CAD build for the part. Positions are in the model's coordinates, mm. A direction names the side the tool comes from. Round coordinates to 2 decimals unless told otherwise and drop trailing zeros. Write each loop counter-clockwise with the first axis right and the second up, starting at its lowest first coordinate (ties: lowest second). Pieces come first, ordered by that corner, then holes. Notation, with made-up numbers: (12.25, 78.25) - (24.25, 78.25) arc R16 cw to (24.25, 103.25) - close; hole circle Ø9 at (41.25, -9). An arc over 180 degrees is marked (long way). Answer in a Markdown table with one row per item.
```python
from build123d import *
from build123d.topology import SkipClean

# Parameters (mm, degrees)
CROQUIS1_R                        = 35
CROQUIS1_R_2                      = 4.75
SALIENTE_EXTRUIR1_DEPTH           = 3
CROQUIS2_R                        = 1.95
SALIENTE_EXTRUIR2_DEPTH           = 5
SALIENTE_EXTRUIR3_START           = 1
CROQUIS5_R                        = 2.25
SALIENTE_EXTRUIR3_DEPTH           = 4
SALIENTE_EXTRUIR3_DRAFT           = 4
SALIENTE_EXTRUIR3_PROFILE_2_DEPTH = 4
SALIENTE_EXTRUIR3_PROFILE_2_DRAFT = 4
CROQUIS3_W                        = 1
CROQUIS3_H                        = 6.840682912
CORTAR_EXTRUIR1_DEPTH             = 4
CROQUIS6_W                        = 5.727241663
CROQUIS6_H                        = 1.622786798
CROQUIS6_W_2                      = 5.017003251
CROQUIS6_H_2                      = 0.546869116
CROQUIS6_W_3                      = 4.668475527
CROQUIS6_H_3                      = 1.179349449
CROQUIS6_W_4                      = 4.588943699
CROQUIS6_H_4                      = 1.521824685
CORTAR_EXTRUIR2_DEPTH             = 4
SALIENTE_EXTRUIR4_START           = 35
SALIENTE_EXTRUIR4_DEPTH           = 35
CROQUIS9_W                        = 86.6
CROQUIS9_H                        = 71.3
SALIENTE_EXTRUIR5_DEPTH           = 3
CROQUIS10_W                       = 86.6
CROQUIS10_H                       = 71.3
CROQUIS10_W_2                     = 80.6
CROQUIS10_H_2                     = 65.3
SALIENTE_EXTRUIR6_DEPTH           = 32
CORTAR_EXTRUIR3_REACH             = 106.595
CROQUIS11_W                       = 40
CROQUIS11_H                       = 3
CROQUIS12_R                       = 2.5
CROQUIS12_R_2                     = 1.59
SALIENTE_EXTRUIR7_DEPTH           = 5
CROQUIS13_W                       = 14
CROQUIS13_H                       = 14
CROQUIS13_W_2                     = 11
CROQUIS13_H_2                     = 11
CORTAR_EXTRUIR4_DEPTH             = 3


with BuildPart() as part:
    # Croquis1 → Saliente-Extruir1 (new body)
    with BuildSketch(Plane(origin=(0, 0, 0), x_dir=(1, 0, 0), z_dir=(0, 1, 0))):
        with Locations(Location((0, 0, 0), (0, 0, 270))):
            Circle(CROQUIS1_R)
        with Locations(Location((0, 0, 0), (0, 0, 270))):
            Circle(CROQUIS1_R_2, mode=Mode.SUBTRACT)
    extrude(amount=SALIENTE_EXTRUIR1_DEPTH)

    # Croquis2 → Saliente-Extruir2 (add)
    with BuildSketch(Plane.XZ):
        with Locations(Location((-17.5, 8, 0), (0, 0, 90))):
            Circle(CROQUIS2_R)
        with Locations(Location((17.5, 8, 0), (0, 0, 90))):
            Circle(CROQUIS2_R)
    extrude(amount=SALIENTE_EXTRUIR2_DEPTH)


with BuildPart() as saliente_extruir3_tool:
    # Croquis5 → Saliente-Extruir3 (with draft: the straight prism first)
    with BuildSketch(Plane.XZ.offset(SALIENTE_EXTRUIR3_START)):
        with Locations((-17.5, 8)):
            Circle(CROQUIS5_R)
    extrude(amount=SALIENTE_EXTRUIR3_DEPTH)
    # Saliente-Extruir3: the draft: its side faces are tilted about the plane it starts from
    saliente_extruir3_sides = [saliente_extruir3_tool.faces().sort_by_distance(p)[0] for p in [
        (-19.75, -3, 8),
    ]]
    draft(saliente_extruir3_sides, Plane.XZ.offset(SALIENTE_EXTRUIR3_START), SALIENTE_EXTRUIR3_DRAFT)


with BuildPart() as part_1:
    add(part.part)

    # Saliente-Extruir3: add saliente_extruir3_tool
    add(saliente_extruir3_tool.part)


with BuildPart() as saliente_extruir3_profile_2_tool:
    # Croquis5 → Saliente-Extruir3 profile 2 (with draft: the straight prism first)
    with BuildSketch(Plane.XZ.offset(SALIENTE_EXTRUIR3_START)):
        with Locations((17.5, 8)):
            Circle(CROQUIS5_R)
    extrude(amount=SALIENTE_EXTRUIR3_PROFILE_2_DEPTH)
    # Saliente-Extruir3 profile 2: the draft: its side faces are tilted about the plane it starts from
    saliente_extruir3_profile_2_sides = [saliente_extruir3_profile_2_tool.faces().sort_by_distance(p)[0] for p in [
        (15.25, -3, 8),
    ]]
    draft(saliente_extruir3_profile_2_sides, Plane.XZ.offset(SALIENTE_EXTRUIR3_START), SALIENTE_EXTRUIR3_PROFILE_2_DRAFT)


with BuildPart() as part_2:
    add(part_1.part)

    # Saliente-Extruir3 profile 2: add saliente_extruir3_profile_2_tool
    add(saliente_extruir3_profile_2_tool.part)

    # Croquis3 → Cortar-Extruir1 (cut)
    with BuildSketch(Plane.XZ.offset(5)):
        with Locations((-17.5, 7.675365729)):
            Rectangle(CROQUIS3_W, CROQUIS3_H)
        with Locations((17.5, 7.675365729)):
            Rectangle(CROQUIS3_W, CROQUIS3_H)
    extrude(amount=-CORTAR_EXTRUIR1_DEPTH, mode=Mode.SUBTRACT)

    # Croquis6 → Cortar-Extruir2 (cut)
    with BuildSketch(Plane.XZ.offset(1)):
        with Locations((-17.258839661, 10.696201081)):
            Rectangle(CROQUIS6_W, CROQUIS6_H)
        with Locations((-17.417509945, 5.84175776)):
            Rectangle(CROQUIS6_W_2, CROQUIS6_H_2)
        with Locations((17.632507556, 10.474482406)):
            Rectangle(CROQUIS6_W_3, CROQUIS6_H_3)
        with Locations((17.310781188, 5.354279976)):
            Rectangle(CROQUIS6_W_4, CROQUIS6_H_4)
    extrude(amount=CORTAR_EXTRUIR2_DEPTH, mode=Mode.SUBTRACT)

    # Croquis7 → Saliente-Extruir4 (add)
    with SkipClean():  # the faces are left unmerged after this step: merging them gives an invalid solid
        with BuildSketch(Plane.XZ.offset(SALIENTE_EXTRUIR4_START)):
            with BuildLine():
                Line((-22.651194874, 22.651194874), (-24.748737342, 24.748737342))
                ThreePointArc((-24.748737342, 24.748737342), (-15.674335611, 31.294012257), (-4.998139738, 34.641284606))
                Line((-4.998139738, 34.641284606), (-4.998139738, 31.641284606))
                ThreePointArc((-4.998139738, 31.641284606), (-14.537086186, 28.545154562), (-22.651194874, 22.651194874))
            make_face()
            with BuildLine():
                Line((22.651200534, 22.651200534), (24.748737342, 24.748737342))
                ThreePointArc((24.748737342, 24.748737342), (15.675128347, 31.293615184), (4.999894801, 34.641031335))
                Line((4.999894801, 34.641031335), (4.999894801, 31.641031335))
                ThreePointArc((4.999894801, 31.641031335), (14.537881979, 28.544766366), (22.651200534, 22.651200534))
            make_face()
        extrude(amount=-SALIENTE_EXTRUIR4_DEPTH)

    # Croquis9 → Saliente-Extruir5 (add)
    with SkipClean():  # the faces are left unmerged after this step: merging them gives an invalid solid
        with BuildSketch(Plane.XZ):
            with Locations((0, -51.65)):
                Rectangle(CROQUIS9_W, CROQUIS9_H)
        extrude(amount=SALIENTE_EXTRUIR5_DEPTH)

    # Croquis10 → Saliente-Extruir6 (add)
    with SkipClean():  # the faces are left unmerged after this step: merging them gives an invalid solid
        with BuildSketch(Plane.XZ.offset(3)):
            with Locations((0, -51.65)):
                Rectangle(CROQUIS10_W, CROQUIS10_H)
            with Locations((0, -51.65)):
                Rectangle(CROQUIS10_W_2, CROQUIS10_H_2, mode=Mode.SUBTRACT)
        extrude(amount=SALIENTE_EXTRUIR6_DEPTH)

    # Cortar-Extruir3: up to this face of the body (flat: up to its plane)
    cortar_extruir3_end = Plane(part_2.part.faces().sort_by_distance((1.0887e-05, 0, 5.820345138))[0])
    # Croquis11 → Cortar-Extruir3 (cut, up to the picked face)
    with BuildSketch(Plane.XZ.offset(35), mode=Mode.PRIVATE) as cortar_extruir3_sk1:
        with Locations((0, -17.5)):
            Rectangle(CROQUIS11_W, CROQUIS11_H)
    cortar_extruir3_tool1 = split(extrude(cortar_extruir3_sk1.sketch, amount=-CORTAR_EXTRUIR3_REACH, mode=Mode.PRIVATE), bisect_by=cortar_extruir3_end, keep=Keep.BOTH, mode=Mode.PRIVATE)
    add(cortar_extruir3_tool1.solids().sort_by(Axis((0, -35, -17.5), (0, 1, 0)))[0], mode=Mode.SUBTRACT)

    # Croquis12 → Saliente-Extruir7 (add)
    # profile 1 of 4: a face of its own
    with SkipClean():  # the faces are left unmerged after this step: merging them gives an invalid solid
        with BuildSketch(Plane.XZ.offset(3)):
            with Locations(Location((31.8, -42.7, 0), (0, 0, 270))):
                Circle(CROQUIS12_R)
            with Locations(Location((31.8, -42.7, 0), (0, 0, 270))):
                Circle(CROQUIS12_R_2, mode=Mode.SUBTRACT)
        # profile 2 of 4: a face of its own
        with BuildSketch(Plane.XZ.offset(3)):
            with Locations(Location((31.8, -70.6, 0), (0, 0, 270))):
                Circle(CROQUIS12_R)
            with Locations(Location((31.8, -70.6, 0), (0, 0, 270))):
                Circle(CROQUIS12_R_2, mode=Mode.SUBTRACT)
        # profile 3 of 4: a face of its own
        with BuildSketch(Plane.XZ.offset(3)):
            with Locations(Location((-19, -27.5, 0), (0, 0, 270))):
                Circle(CROQUIS12_R)
            with Locations(Location((-19, -27.5, 0), (0, 0, 270))):
                Circle(CROQUIS12_R_2, mode=Mode.SUBTRACT)
        # profile 4 of 4: a face of its own
        with BuildSketch(Plane.XZ.offset(3)):
            with Locations(Location((-20.1, -75.3, 0), (0, 0, 270))):
                Circle(CROQUIS12_R)
            with Locations(Location((-20.1, -75.3, 0), (0, 0, 270))):
                Circle(CROQUIS12_R_2, mode=Mode.SUBTRACT)
        extrude(amount=SALIENTE_EXTRUIR7_DEPTH)

    # Croquis13 → Cortar-Extruir4 (cut)
    with SkipClean():  # the faces are left unmerged after this step: merging them gives an invalid solid
        with BuildSketch(Plane(origin=(-40.3, 0, 0), x_dir=(0, 0, -1), z_dir=(1, 0, 0))):
            with Locations((40.6, -15)):
                Rectangle(CROQUIS13_W, CROQUIS13_H)
            with Locations((70.8, -13.5)):
                Rectangle(CROQUIS13_W_2, CROQUIS13_H_2)
        extrude(amount=-CORTAR_EXTRUIR4_DEPTH, mode=Mode.SUBTRACT)


solid = part_2.part
```
Q1. Saw through at C-C on x = 0. List the corners of the cut face in (y, z), then the cut area to 3 significant figures.
Computed:
| item | result |
|---|---|
| outline | (-35, -87.3) - (0, -87.3) - (0, -35) - (3, -35) - (3, -4.75) - (0, -4.75) - (0, -19) - (-3, -19) - (-3, -84.3) - (-35, -84.3) - close; (0, 4.75) - (3, 4.75) - (3, 35) - (0, 35) - close |
| area | 482 mm2 |
Q2. Saw through at D-D on z = -49. List the corners of the cut face in (x, y).
Computed:
| item | result |
|---|---|
| outline | (-43.3, -35) - (-40.3, -35) - (-40.3, -3) - (40.3, -3) - (40.3, -35) - (43.3, -35) - (43.3, 0) - (-43.3, 0) - close |
Q3. Flat gauge pins, fed straight in: pin 1 (10 mm diameter, centred on x = 11.5, z = 3, fed in from -Y); pin 2 (0.7 mm diameter, centred on x = -16, z = 7, fed in from -Y); pin 3 (1 mm diameter, centred on x = 25.5, z = -22, fed in from -Y). Where does each tip first touch, or does it go through?
Computed:
| item | result |
|---|---|
| pin 1 | stops at y = 0 |
| pin 2 | stops at y = -5 |
| pin 3 | stops at y = -3 |
Q4. Saw through at B-B on y = -15. List the corners of the cut face in (x, z), then the cut area to 3 significant figures.
Computed:
| item | result |
|---|---|
| outline | (-43.3, -87.3) - (43.3, -87.3) - (43.3, -16) - (20, -16) - (20, -19) - (40.3, -19) - (40.3, -84.3) - (-40.3, -84.3) - (-40.3, -76.3) - (-43.3, -76.3) - close; (-43.3, -65.3) - (-40.3, -65.3) - (-40.3, -47.6) - (-43.3, -47.6) - close; (-43.3, -33.6) - (-40.3, -33.6) - (-40.3, -19) - (-20, -19) - (-20, -16) - (-43.3, -16) - close; (-24.75, 24.75) - (-22.65, 22.65) arc R32.03 cw to (-5, 31.64) - (-5, 34.64) arc R35 ccw to start; (5, 31.64) arc R32.03 cw to (22.65, 22.65) - (24.75, 24.75) arc R35 ccw to (5, 34.64) - close |
| area | 843 mm2 |
Q5. Pull direction Z, two halves, no side cores. Call faces 5 (the cylindrical face through (18.687, -0.493, 6.453)), 6 (the flat face through (5, -18, 33)), 7 (the flat face through (-32, -17, -16)): released by +Z, released by -Z, zero draft, split by the parting line, or undercut.
Computed:
| item | result |
|---|---|
| face 5 | undercut |
| face 6 | zero draft |
| face 7 | undercut |
Q6. Drill centre lines: line 1 (X direction, y = -5, z = -75); line 2 (X direction, y = -5.65, z = -42.7); line 3 (X direction, y = -28.5, z = -61). Where is each one in solid material? Low to high.
Computed:
| item | result |
|---|---|
| line 1 | x = -43.3 to -40.3, -22.58 to -21.66, -18.54 to -17.62, 40.3 to 43.3 |
| line 2 | x = -43.3 to -40.3, 29.3 to 30.21, 33.39 to 34.3, 40.3 to 43.3 |
| line 3 | x = -43.3 to -40.3, 40.3 to 43.3 |
Q7. Saw through at A-A on z = 0. List the corners of the cut face in (x, y), then the cut area to 4 significant figures.
Computed:
| item | result |
|---|---|
| outline | (-35, 0) - (-4.75, 0) - (-4.75, 3) - (-35, 3) - close; (4.75, 0) - (35, 0) - (35, 3) - (4.75, 3) - close |
| area | 181.5 mm2 |
Q8. 3-axis set-ups, long thin cutter, end or side, ignore diameter. For faces 1 (the flat face through (-42, -15, -47.6)), 2 (the flat face through (30, -8, -71)), 3 (the cylindrical face through (-16.313, -0.493, 6.453)), 4 (the cylindrical face through (-18.759, -5.465, -76.155)): which of +Z, -Z, +X, -X, +Y, -Y reach the whole face in a straight line?
Computed:
| item | result |
|---|---|
| face 1 | -X |
| face 2 | -X, -Y |
| face 3 | none |
| face 4 | -Y |
